Source: three-view drawing plus pictorial views. Frame: mm from the lowest corner of the part. A direction names the side the tool comes from. Give positions to 0.01 mm unless a question says otherwise; leave off trailing zeros. Loops run counter-clockwise (first coordinate to the right, second up) from the corner with the lowest first, then second, coordinate; pieces in that order, holes last. Notation, with made-up numbers: (79.25, 9) - (87.25, 9) arc R23 ccw to (87.25, 29) - close; hole circle Ø3 at (-34, -31). An arc over 180 degrees is marked (long way). Write each question's results on one line, items separated by ' | '. Start each with the question number.
(1) Pull-direction query (X, two-part tool) for the marked faces 3, 4 and 5; classes: pulls with the +X half, pulls with the -X half, needs draft (parallel to the pull), parting line crosses it, or undercut.
(2) Cut plane A-A on z = 14.5. Return the cut outline in (x, y), then the cut area to 3 significant figures.
(3) Cut plane B-B on y = 61.5. Return the cut outline in (x, z).
(4) Cut plane C-C on x = 19.5. Return the cut outline in (y, z).
(5) Reachability of the marked faces 1 and 2 from +Z, -Z, +X, -X, +Y, -Y: full face, straight path, thin tool, end or side. Return the list, or none.
(6) Material intervals for line 1 along X through (y, z) = (35.5, 31); line 2 along Z through (x, y) = (9, 53), sorted ascending. Write a range as [from, to].
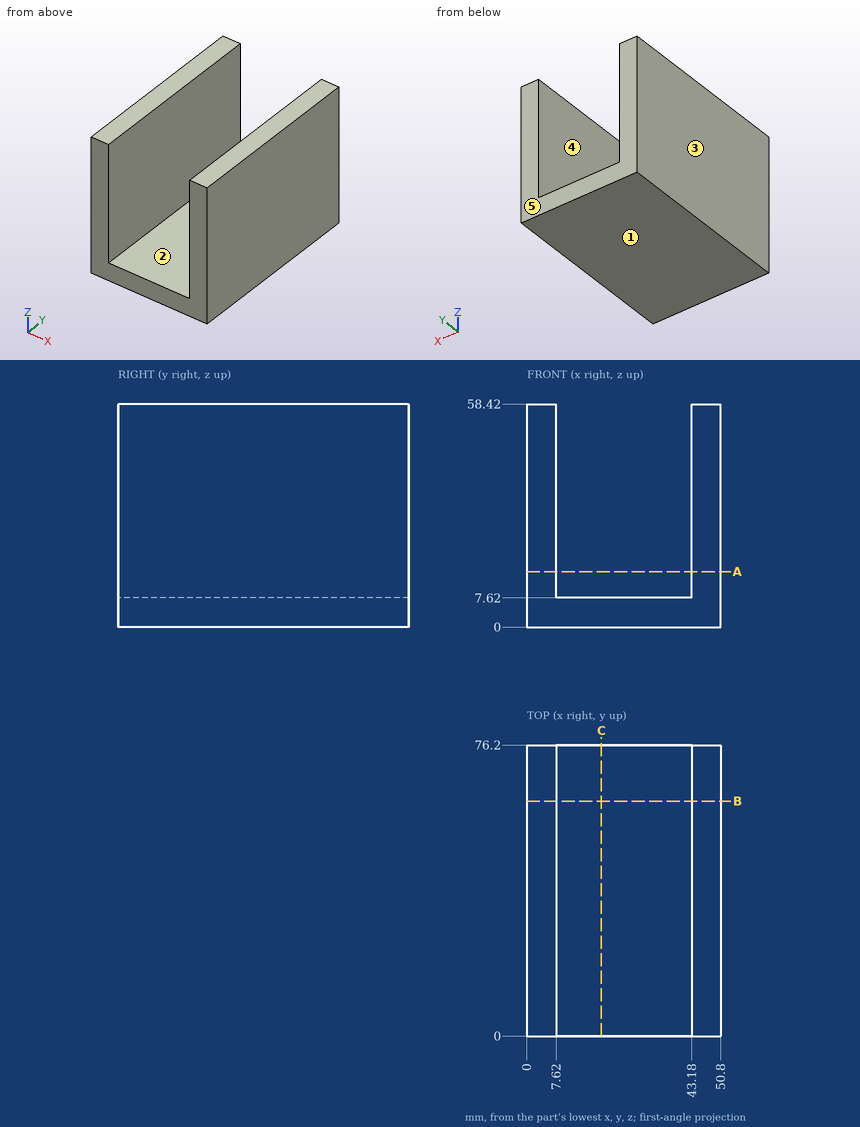
Ans:
1) face 3: pulls with the -X half | face 4: undercut | face 5: needs draft
2) outline: (0, 0) - (7.62, 0) - (7.62, 76.2) - (0, 76.2) - close; (43.18, 0) - (50.8, 0) - (50.8, 76.2) - (43.18, 76.2) - close | area: 1,160 mm^2
3) outline: (0, 0) - (50.8, 0) - (50.8, 58.42) - (43.18, 58.42) - (43.18, 7.62) - (7.62, 7.62) - (7.62, 58.42) - (0, 58.42) - close
4) outline: (0, 0) - (76.2, 0) - (76.2, 7.62) - (0, 7.62) - close
5) face 1: -Z, +X, -X, +Y, -Y | face 2: +Z, +Y, -Y
6) line 1: [0, 7.62], [43.18, 50.8] | line 2: [0, 7.62]
